```python
from build123d import *

# Parameters (mm, degrees)
SKETCH1_R           = 12.5
BOSS_EXTRUDE1_DEPTH = 52
SKETCH2_R           = 3.5
BOSS_EXTRUDE2_DEPTH = 2.5
BOSS_EXTRUDE3_DEPTH = 9.5
SKETCH4_R           = 1.5
CUT_EXTRUDE1_DEPTH  = 8


with BuildPart() as part:
    # Sketch1 → Boss-Extrude1 (new body)
    with BuildSketch(Plane(origin=(0, 0, 0), x_dir=(1, 0, 0), z_dir=(0, 1, 0))):
        with Locations(Location((0, 0, 0), (0, 0, 90))):
            Circle(SKETCH1_R)
    extrude(amount=BOSS_EXTRUDE1_DEPTH)

    # Sketch2 → Boss-Extrude2 (add)
    with BuildSketch(Plane(origin=(0, 52, 0), x_dir=(1, 0, 0), z_dir=(0, 1, 0))):
        with Locations(Location((0, 0, 0), (0, 0, 270))):
            Circle(SKETCH2_R)
    extrude(amount=BOSS_EXTRUDE2_DEPTH)

    # Sketch3 → Boss-Extrude3 (add)
    with BuildSketch(Plane(origin=(0, 54.5, 0), x_dir=(1, 0, 0), z_dir=(0, 1, 0))):
        with BuildLine():
            ThreePointArc((-1.322875656, 1.5), (-1.870828693, -0.707106781), (0, -2))
            Line((0, -2), (0, 1.5))
            Line((0, 1.5), (-1.322875656, 1.5))
        make_face()
        with BuildLine():
            Line((0, 1.5), (0, -2))
            ThreePointArc((0, -2), (1.870828693, -0.707106781), (1.322875656, 1.5))
            Line((1.322875656, 1.5), (0, 1.5))
        make_face()
    extrude(amount=BOSS_EXTRUDE3_DEPTH)

    # Sketch4 → Cut-Extrude1 (cut)
    with BuildSketch(Plane(origin=(0, 52, 0), x_dir=(1, 0, 0), z_dir=(0, 1, 0))):
        with BuildLine():
            ThreePointArc((-7, 0), (-8.5, 1.5), (-10, 0))
            Line((-10, 0), (-7, 0))
        make_face()
        with BuildLine():
            Line((-7, 0), (-10, 0))
            ThreePointArc((-10, 0), (-8.5, -1.5), (-7, 0))
        make_face()
        with Locations(Location((8.5, 0, 0), (0, 0, 270))):
            Circle(SKETCH4_R)
    extrude(amount=-CUT_EXTRUDE1_DEPTH, mode=Mode.SUBTRACT)


solid = part.part
```
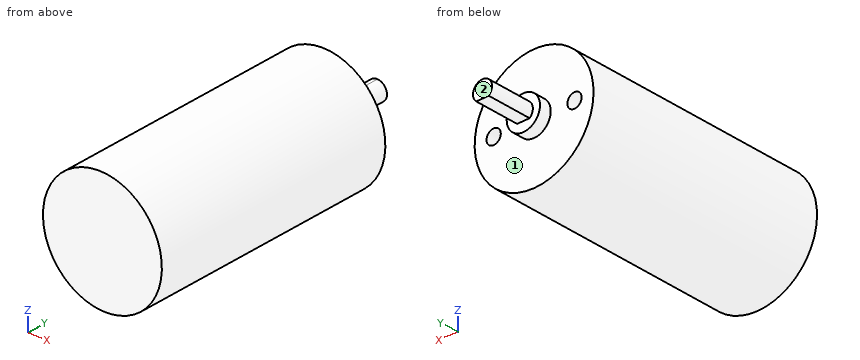
Input: part model. Units: mm. Frame: model coordinates. Face numbers are marked on the shaded views. A direction names the side the tool comes from. Coordinates: 2 decimals unless noted, no trailing zeros. Write each loop counter-clockwise with the first axis right and the second up, starting at its lowest first coordinate (ties: lowest second). Pieces come first, ordered by that corner, then holes. Notation, with made-up numbers: M 64.5,88 L 95.5,88 A15 cw 95.5,97 Z; hole C 16.25,51 d6. An arc over 180 degrees is marked long. Use one line per item in the form item = value.
Q1. Section A-A (z = 0). Return loops of the section in (x, y).
Answer below:
outline = M -12.5,0 L 12.5,0 L 12.5,52 L 10,52 L 10,44 L 7,44 L 7,52 L 3.5,52 L 3.5,54.5 L 2,54.5 L 2,64 L -2,64 L -2,54.5 L -3.5,54.5 L -3.5,52 L -7,52 L -7,44 L -10,44 L -10,52 L -12.5,52 Z
Q2. Section B-B (x = -8.5). Return loops of the section in (y, z), plus the area to 3 significant figures.
Answer below:
outline = M 0,-9.17 L 52,-9.17 L 52,-1.5 L 44,-1.5 L 44,1.5 L 52,1.5 L 52,9.17 L 0,9.17 Z
area = 929 mm²
Q3. Section C-C (y = 36.5). Return loops of the section in (x, z), plus the area to 3 significant figures.
Answer below:
outline = C 0,0 d25
area = 491 mm²
Q4. Material intervals for probe 1 along Y at (x, z) = (6.5, -10.5); probe 2 along Z at (x, y) = (-8.5, 48.25); probe 3 along X at (y, z) = (13.5, 0.5), sorted ascending. Write a range as from..to.
Answer below:
probe_1 = 0..52
probe_2 = -9.17..-1.5, 1.5..9.17
probe_3 = -12.49..12.49
Q5. First-contact query: pin 1 (1 mm diameter, centred on y = 41.5, z = -5.5, fed in from -X); pin 2 (5 mm diameter, centred on x = -8.5, z = 0, fed in from +Y); pin 3 (1.3 mm diameter, centred on x = -0.5, y = 60, fed in from -Z). Flat tips, straight axial feed; report the tip coordinate or a pass-through.
Answer below:
pin_1 = -11.46
pin_2 = 52
pin_3 = -1.5
Q6. Set-up query: the marked faces 1 and 2. Return all of +Z, -Z, +X, -X, +Y, -Y with unobstructed straight access to the full face (end or side cutting, diameter ignored); none if empty.
Answer below:
face_1 = +Y
face_2 = +Z, -Z, +X, -X, +Y
Q7. Section D-D (z = -10). Return loops of the section in (x, y).
Answer below:
outline = M -7.5,0 L 7.5,0 L 7.5,52 L -7.5,52 Z
